Autodesk Inventor part; units mm, degrees
ref_plane "YZ Plane" through (0, 0, 0) normal (1, 0, 0) x (0, 1, 0)
ref_plane "XZ Plane" through (0, 0, 0) normal (0, 1, 0) x (-1, 0, 0)
ref_plane "XY Plane" through (0, 0, 0) normal (0, 0, 1) x (1, 0, 0)
sketch "Эскиз1" plane through (0, 0, 0) normal (0, 0, 1) x (1, 0, 0)
  circle A0 centre (0, 0) radius 6
  circle A1 centre (18, 0) radius 4
  line L0 (0, 0) -> (18, 0)
  line L1 (0, 0) -> (18, 0) construction
  line L2 (1, -8.9443) -> (18.7778, -6.9567)
  line L3 (18.7778, 6.9567) -> (1, 8.9443)
  arc A2 (1, 8.9443) -> (1, -8.9443) centre (0, 0) ccw
  arc A3 (18.7778, -6.9567) -> (18.7778, 6.9567) centre (18, 0) ccw
  point P0 (9, 0)
  dimension "d0" = 12
  dimension "d1" = 8
  dimension "d2" = 18
  dimension "d4" = 9
  dimension "d7" = 7
extrude "Выдавливание1" add sketch "Эскиз1" along normal blind 6
properties part number "Крепление петли"
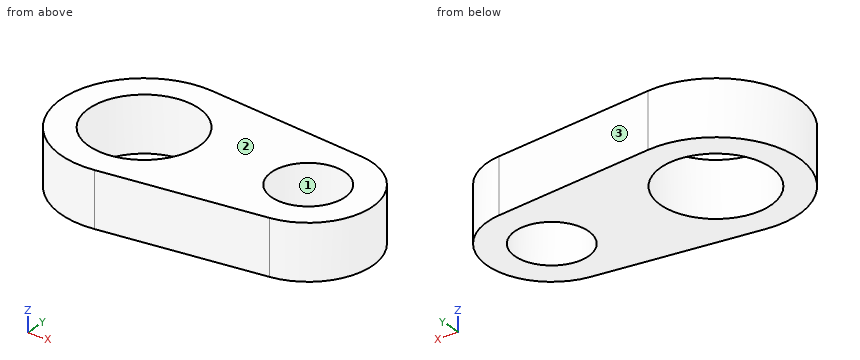
Read the model definition and answer for the solid it produces. Units are mm, in the model's axes. Face numbers are marked on the shaded views. Round coordinates to 2 decimals unless told otherwise and drop trailing zeros. Write each loop counter-clockwise with the first axis right and the second up, starting at its lowest first coordinate (ties: lowest second). Pieces come first, ordered by that corner, then holes. Notation, with made-up numbers: (-5, 76.25) - (39, 76.25) arc R25 ccw to (39, 94.25) - close; hole circle Ø7 at (10, 58.25). An arc over 180 degrees is marked (long way). One line per item, written item: value.
Q1. For a pull along X with two mould halves and no side action, classify the marked faces 1, 2 and 3 as pulls with the +X half, pulls with the -X half, needs draft (parallel to the pull), parting line crosses it, or undercut.
The answers:
face 1: undercut
face 2: needs draft
face 3: pulls with the +X half
Q2. Find section B-B (y = 2.5). Determine the outline of the cut face in (x, z), and give its area (3 significant figures).
The answers:
outline: (-8.65, 0) - (-5.45, 0) - (-5.45, 6) - (-8.65, 6) - close; (5.45, 0) - (14.88, 0) - (14.88, 6) - (5.45, 6) - close; (21.12, 0) - (24.54, 0) - (24.54, 6) - (21.12, 6) - close
area: 96.2 mm2
Q3. Each of these flat-tipped pins is pushed along its axis until it touches: P1, Ø7, axis at x = 0, y = 0, coming from the +Z side; P2, Ø1.5, axis at x = 20, z = 1.5, coming from the -Y side; P3, Ø1.5, axis at y = 5, z = 2.5, coming from the +X side; P4, Ø2, axis at y = 1.5, z = 0.5, coming from the -X side. Where does it stop, or does it pass through?
The answers:
P1: passes through
P2: stops at y = -6.89
P3: stops at x = 23.56
P4: stops at x = -8.99
Q4. Find section D-D (x = 18). Determine the outline of the cut face in (y, z).
The answers:
outline: (-7.04, 0) - (-4, 0) - (-4, 6) - (-7.04, 6) - close; (4, 0) - (7.04, 0) - (7.04, 6) - (4, 6) - close
Q5. Find section C-C (z = 2.45). Determine the outline of the cut face in (x, y), and give its area (3 significant figures).
The answers:
outline: (1, -8.94) - (18.78, -6.96) arc R7 ccw to (18.78, 6.96) - (1, 8.94) arc R9 ccw (long way) to start; hole circle Ø12 at (0, 0); hole circle Ø8 at (18, 0)
area: 331 mm2
Q6. Find section A-A (x = 0). Determine the outline of the cut face in (y, z), and give its area (3 significant figures).
The answers:
outline: (-9, 0) - (-6, 0) - (-6, 6) - (-9, 6) - close; (6, 0) - (9, 0) - (9, 6) - (6, 6) - close
area: 36.0 mm2
Q7. Straight lines are drawn through the part: line 1 (Y direction, x = 0, z = 2.2); line 2 (X direction, y = 3.5, z = 4.85); line 3 (X direction, y = -3, z = 3.2). For each, find the intervals that lie inside material, in ascending order. Write a range as from..to.
The answers:
line 1: y = -9..-6, 6..9
line 2: x = -8.29..-4.87, 4.87..16.06, 19.94..24.06
line 3: x = -8.49..-5.2, 5.2..15.35, 20.65..24.32
